Answer from the drawing. Dimensions are ordinates in mm from the lowest x, y and z of the part. A direction names the side the tool comes from. Round coordinates to 2 decimals unless told otherwise and drop trailing zeros. Loops run counter-clockwise (first coordinate to the right, second up) from the corner with the lowest first, then second, coordinate; pieces in that order, holes last. Notation, with made-up numbers: M 16.5,-39.5 L 75.5,-39.5 A21 ccw 75.5,-13.5 Z; hole C 1.25,39.5 d2. An arc over 180 degrees is marked long. One line per item, written item: value.
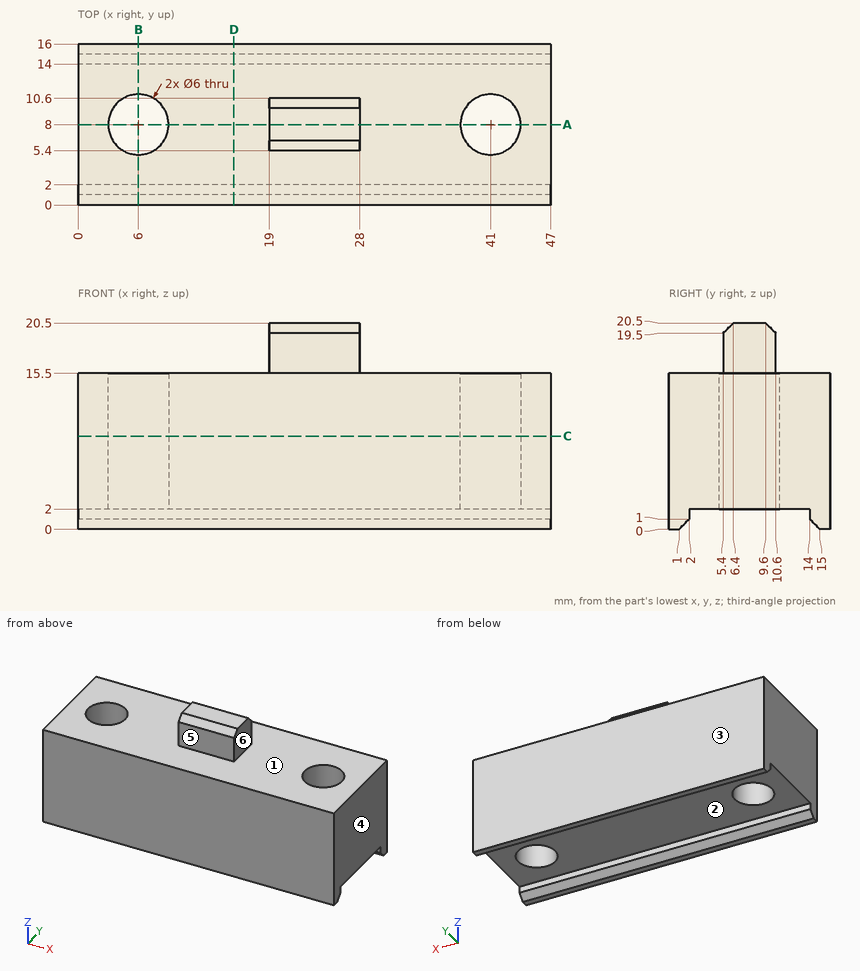
1) Find section D-D (x = 15.5). Give the vertices of the cut face in (y, z), then the cut area to 3 significant figures.
Check values:
outline: M 0,0 L 1,0 L 2,1 L 2,2 L 14,2 L 14,1 L 15,0 L 16,0 L 16,15.5 L 0,15.5 Z
area: 223 mm2
2) Each of these flat-tipped pins is pushed along its axis until it touches: pin 1 (3 mm diameter, centred on x = 29, z = 18, fed in from -Y); pin 2 (5 mm diameter, centred on x = 11.5, z = 6.5, fed in from -Y); pin 3 (2.5 mm diameter, centred on y = 7, z = 17.5, fed in from +X); pin 4 (3.5 mm diameter, centred on x = 25, y = 7.5, fed in from -Z). Where does it stop, or does it pass through?
Check values:
pin 1: y = 5.4
pin 2: y = 0
pin 3: x = 28
pin 4: z = 2
3) Find section A-A (y = 8). Give the vertices of the cut face in (x, z), then the cut area to 4 significant figures.
Check values:
outline: M 0,2 L 3,2 L 3,15.5 L 0,15.5 Z; M 9,2 L 38,2 L 38,15.5 L 28,15.5 L 28,20.5 L 19,20.5 L 19,15.5 L 9,15.5 Z; M 44,2 L 47,2 L 47,15.5 L 44,15.5 Z
area: 517.5 mm2
4) For the marked faces 4, 5 and 6, determine the directions among +Z, -Z, +X, -X, +Y, -Y from which every point of the face is accessible in a straight line to the end or side of a thin tool.
Check values:
face 4: +Z, -Z, +X, +Y, -Y
face 5: +Z, +X, -X, -Y
face 6: +Z, +X, +Y, -Y
5) Find section B-B (x = 6). Give the vertices of the cut face in (y, z).
Check values:
outline: M 0,0 L 1,0 L 2,1 L 2,2 L 5,2 L 5,15.5 L 0,15.5 Z; M 11,2 L 14,2 L 14,1 L 15,0 L 16,0 L 16,15.5 L 11,15.5 Z
6) The mould has two halves that part along Y. Classify the marked faces 1, 2 and 3: +Y half, -Y half, draft (parallel to the pull), parting line (faces both ways), or undercut.
Check values:
face 1: draft
face 2: undercut
face 3: +Y half
7) Find the intervals of material crossed by probe 1 along Y at (x, z) = (6, 4.25); probe 2 along Y at (x, z) = (40.5, 1.25); probe 3 along X at (y, z) = (8.5, 6.75), in increasing order. Write a range as from..to.
Check values:
probe 1: 0..5, 11..16
probe 2: 0..2, 14..16
probe 3: 0..3.04, 8.96..38.04, 43.96..47
8) Find section C-C (z = 9.25). Give the vertices of the cut face in (x, y).
Check values:
outline: M 0,0 L 47,0 L 47,16 L 0,16 Z; hole C 6,8 d6; hole C 41,8 d6
